from build123d import *

# Parameters (mm, degrees)
SKETCH1_W                  = 12.7
SKETCH1_H                  = 12.7
BOSS_EXTRUDE1_DEPTH        = 101.6
TAP_DRILL_FOR_10_24_TAP1_D = 3.7973
TAP_DRILL_FOR_10_24_TAP2_D = 3.7973


with BuildPart() as part:
    # Sketch1 → Boss-Extrude1 (new body)
    with BuildSketch(Plane(origin=(0, 0, 0), x_dir=(1, 0, 0), z_dir=(0, 1, 0))):
        Rectangle(SKETCH1_W, SKETCH1_H)
    extrude(amount=BOSS_EXTRUDE1_DEPTH)

    # Tap Drill for #10-24 Tap1 (through all)
    with Locations(Plane(origin=(6.35, 0, 0), x_dir=(0, 0, -1), z_dir=(1, 0, 0))):
        with Locations((3.175, 82.55), (3.175, 12.7), (3.175, 57.15)):
            Hole(TAP_DRILL_FOR_10_24_TAP1_D / 2)

    # Tap Drill for #10-24 Tap2 (through all)
    with Locations(Plane.XY.offset(6.35)):
        with Locations((2.38125, 92.075), (2.38125, 6.35), (2.38125, 34.925), (2.38125, 63.5)):
            Hole(TAP_DRILL_FOR_10_24_TAP2_D / 2)


solid = part.part
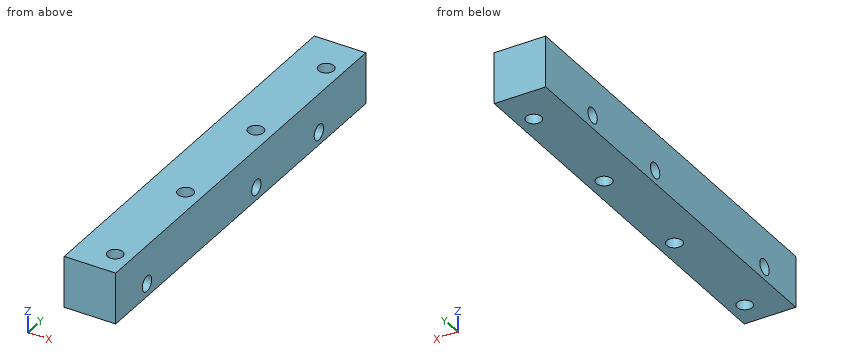
Design review of the part built by this model. Coordinates are the model's own, in mm. Give positions to 0.01 mm unless a question says otherwise; leave off trailing zeros. Loops run counter-clockwise (first coordinate to the right, second up) from the corner with the lowest first, then second, coordinate; pieces in that order, holes last. Notation, with made-up numbers: (-23, 30.5) -> (3, 30.5) arc R15 cw to (3, 58.5) -> close; hole circle Ø5 at (49.5, 72). An arc over 180 degrees is marked (long way). One line per question, with ' | ' between items. Start each with the question number.
(1) Insertion check: P1, Ø6, axis at x = 2.38, y = 34.92, coming from the +Z side; P2, Ø2.5, axis at x = 2.38, y = 6.35, coming from the -Z side. Each pin has a flat end and moves straight along its axis. Give the tip position at first contact, or say it passes through.
(2) For line 1 (Y direction, x = 2.5, z = 0.5); line 2 (Y direction, x = 1.5, z = -1); line 3 (Y direction, x = -2.25, z = -4), list the stretches that pass through material, from the lowest coordinate up.
(3) We need section B-B (y = 63.5). State the section outline as (x, z) points.
(4) We need section A-A (z = -2.75). State the section outline as (x, y) points (3 decimals), and give its area (3 significant figures).
(5) We need section C-C (x = 2). State the section outline as (y, z) points (3 decimals).
The answers:
1) P1: stops at z = 6.35 | P2: passes through
2) line 1: y = 0 to 4.46, 8.24 to 33.03, 36.82 to 61.61, 65.39 to 90.18, 93.97 to 101.6 | line 2: y = 0 to 4.67, 8.03 to 33.24, 36.61 to 61.82, 65.18 to 90.39, 93.76 to 101.6 | line 3: y = 0 to 10.99, 14.41 to 55.44, 58.86 to 80.84, 84.26 to 101.6
3) outline: (-6.35, -6.35) -> (0.48, -6.35) -> (0.48, 6.35) -> (-6.35, 6.35) -> close; (4.28, -6.35) -> (6.35, -6.35) -> (6.35, 6.35) -> (4.28, 6.35) -> close
4) outline: (-6.35, 0) -> (6.35, 0) -> (6.35, 10.85) -> (-6.35, 10.85) -> close; (-6.35, 14.55) -> (6.35, 14.55) -> (6.35, 55.3) -> (-6.35, 55.3) -> close; (-6.35, 59) -> (6.35, 59) -> (6.35, 80.7) -> (-6.35, 80.7) -> close; (-6.35, 84.4) -> (6.35, 84.4) -> (6.35, 101.6) -> (-6.35, 101.6) -> close; hole circle Ø3.797 at (2.381, 6.35); hole circle Ø3.797 at (2.381, 34.925); hole circle Ø3.797 at (2.381, 63.5); hole circle Ø3.797 at (2.381, 92.075) | area: 1,100 mm^2
5) outline: (0, -6.35) -> (4.49, -6.35) -> (4.49, 6.35) -> (0, 6.35) -> close; (8.21, -6.35) -> (33.065, -6.35) -> (33.065, 6.35) -> (8.21, 6.35) -> close; (36.785, -6.35) -> (61.64, -6.35) -> (61.64, 6.35) -> (36.785, 6.35) -> close; (65.36, -6.35) -> (90.215, -6.35) -> (90.215, 6.35) -> (65.36, 6.35) -> close; (93.935, -6.35) -> (101.6, -6.35) -> (101.6, 6.35) -> (93.935, 6.35) -> close; hole circle Ø3.797 at (12.7, -3.175); hole circle Ø3.797 at (57.15, -3.175); hole circle Ø3.797 at (82.55, -3.175)
